from build123d import *

# Parameters (mm, degrees)
CROQUIS1_R              = 10
CROQUIS1_R_2            = 5.1
SALIENTE_EXTRUIR1_DEPTH = 30
CROQUIS2_OUTSIDE_W      = 35.266
CROQUIS2_OUTSIDE_H      = 35.266
CROQUIS2_OUTSIDE_R      = 8
CORTAR_EXTRUIR1_DEPTH   = 10
CHAFL_N1_SIZE           = 0.5
CROQUIS3_W              = 6
CROQUIS3_H              = 1.2
CHAFL_N2_SIZE           = 1


with BuildPart() as part:
    # Croquis1 → Saliente-Extruir1 (new, symmetric)
    with BuildSketch(Plane.XY):
        Circle(CROQUIS1_R)
        Circle(CROQUIS1_R_2, mode=Mode.SUBTRACT)
    extrude(amount=SALIENTE_EXTRUIR1_DEPTH, both=True)

    # Croquis2 outside → Cortar-Extruir1 (cut)
    with BuildSketch(Plane.XY.offset(30)):
        Rectangle(CROQUIS2_OUTSIDE_W, CROQUIS2_OUTSIDE_H)
        Circle(CROQUIS2_OUTSIDE_R, mode=Mode.SUBTRACT)
    extrude(amount=-CORTAR_EXTRUIR1_DEPTH, mode=Mode.SUBTRACT)

    # Chaflán1
    chafl_n1_edges = [part.edges().sort_by_distance(p)[0] for p in [
        (-8, 0, 30),
        (-5.1, 0, -30),
        (-5.1, 0, 30),
    ]]
    chamfer(chafl_n1_edges, length=CHAFL_N1_SIZE)

    # Croquis3 → Cortar-Revolución1 (revolve, cut)
    with BuildSketch(Plane(origin=(0, 0, 0), x_dir=(1, 0, 0), z_dir=(0, 1, 0))):
        with Locations((10.2, -23.6)):
            Rectangle(CROQUIS3_W, CROQUIS3_H)
    revolve(axis=Axis((0, 0, 0), (0, 0, 1)), mode=Mode.SUBTRACT)

    # Chaflán2
    chafl_n2_edges = [part.edges().sort_by_distance(p)[0] for p in [
        (-10, 0, -30),
    ]]
    chamfer(chafl_n2_edges, length=CHAFL_N2_SIZE)


solid = part.part
Part model, mm, in its own coordinate system. A direction names the side the tool comes from. Give positions to 0.01 mm unless a question says otherwise; leave off trailing zeros. Loops run counter-clockwise (first coordinate to the right, second up) from the corner with the lowest first, then second, coordinate; pieces in that order, holes last.
(1) Band-saw the part on A-A (y = 0). Write the cut outline in (x, z).
Return value:
outline: (-10, -29) - (-9, -30) - (-5.6, -30) - (-5.1, -29.5) - (-5.1, 29.5) - (-5.6, 30) - (-7.5, 30) - (-8, 29.5) - (-8, 24.2) - (-7.2, 24.2) - (-7.2, 23) - (-8, 23) - (-8, 20) - (-10, 20) - close; (5.1, -29.5) - (5.6, -30) - (9, -30) - (10, -29) - (10, 20) - (8, 20) - (8, 23) - (7.2, 23) - (7.2, 24.2) - (8, 24.2) - (8, 29.5) - (7.5, 30) - (5.6, 30) - (5.1, 29.5) - close
(2) Pin check, flat tips, straight feed: pin 1 (4 mm diameter, centred on y = -5, z = -4, fed in from -X); pin 2 (4 mm diameter, centred on x = 4.5, z = -4, fed in from -Y); pin 3 (11.5 mm diameter, centred on x = 0, y = 0, fed in from -Z); pin 4 (3 mm diameter, centred on y = 6, z = 17, fed in from -X). Stop position of each tip, or through.
Return value:
pin 1: stops at x = -9.54
pin 2: stops at y = -9.68
pin 3: stops at z = -30
pin 4: stops at x = -8.93
(3) 3-axis set-ups, long thin cutter, end or side, ignore diameter. For faces 1 (the cylindrical face through (-2.17, -9.76, -4.16)), 2 (the flat face through (7, 3, 24.2)), 3 (the cylindrical face through (-1.73, -7.81, 26.89)): which of +Z, -Z, +X, -X, +Y, -Y reach the whole face in a straight line?
Return value:
face 1: +Z, -Z
face 2: none
face 3: +Z
(4) Pull direction Y, two halves, no side cores. Call faces 4 (the flat face through (0, 8.2, 20)), 5 (the cylindrical face through (6.87, 2.16, 23.59)), 6 (the cylindrical face through (2.4, -4.5, -0.4)): pulls with the +Y half, pulls with the -Y half, needs draft (parallel to the pull), parting line crosses it, or undercut.
Return value:
face 4: needs draft
face 5: parting line crosses it
face 6: undercut
(5) Drill centre lines: line 1 along Y through (x, z) = (0, 7.5); line 2 along X through (y, z) = (-0.25, -18.5); line 3 along Z through (x, y) = (-6.5, -3.75). Where is each one in solid material? Low to high.
Return value:
line 1: y = -10 to -5.1, 5.1 to 10
line 2: x = -10 to -5.09, 5.09 to 10
line 3: z = -30 to 23, 24.2 to 30
(6) Band-saw the part on D-D (z = 22). Write the cut outline in (x, y), and give its area (3 significant figures).
Return value:
outline: circle Ø16 at (0, 0); hole circle Ø10.2 at (0, 0)
area: 119 mm2
(7) Band-saw the part on C-C (z = 10). Write the cut outline in (x, y), and give its area (3 significant figures).
Return value:
outline: circle Ø20 at (0, 0); hole circle Ø10.2 at (0, 0)
area: 232 mm2
